The figure shows three views and two pictorial views of one solid part (mm, origin at its lowest corner). Answer the questions. A direction names the side the tool comes from. Coordinates: 2 decimals unless noted, no trailing zeros. Loops run counter-clockwise (first coordinate to the right, second up) from the corner with the lowest first, then second, coordinate; pieces in that order, holes last. Notation, with made-up numbers: (20.25, 72) -> (44.25, 72) arc R10 ccw to (44.25, 82) -> close; hole circle Ø10 at (-9, 51). An arc over 180 degrees is marked (long way). Answer as a JSON object with one key per item and string values. Group by question number.
1) Section C-C, the plane x = 34 is taken. Give the vertices of the cut face in (y, z).
2) Section D-D, the plane z = 13.75 is taken. Give the vertices of the cut face in (x, y).
3) Which of the six approach directions +Z, -Z, +X, -X, +Y, -Y give full straight-line access (tool end or side, diameter ignored) to the marked faces 1, 2 and 3?
4) Section B-B, the plane z = 4.56 is taken. Give the vertices of the cut face in (x, y), plus the area to 3 significant figures.
5) Section A-A, the plane y = 38.5 is taken. Give the vertices of the cut face in (x, z), plus the area to 3 significant figures.
6) Flat-ended cylindrical pins translate along their axes: P1, Ø8, axis at y = 24.5, z = 19.5, coming from the -X side; P2, Ø8, axis at y = 25.5, z = 11.5, coming from the +X side; P3, Ø12, axis at x = 60, z = 12, coming from the +Y side; P4, Ø1.8, axis at x = 24.81, z = 22.94, coming from the +Y side. Find the tip coordinate at first contact, or state that the pin passes through.
7) Consider probe 1 along Z at (x, y) = (43.19, 63.4); probe 2 along X at (y, z) = (62.65, 22.94); probe 3 along Z at (x, y) = (43, 63). Determine where each line is inside the solid, lowest interval first. Write a range as [from, to].
8) Determine the mould class of the marked faces 4, 5 and 6 for opening direction X: released by +X, released by -X, zero draft, split by the parting line, or undercut.
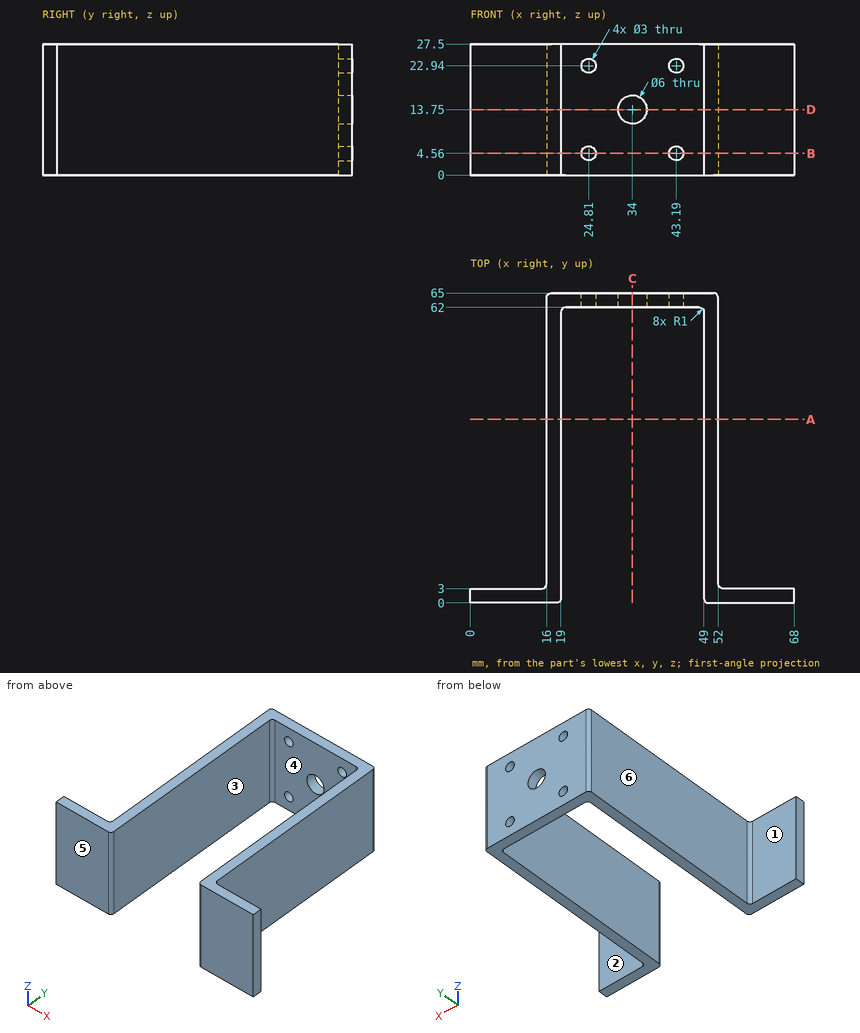
Determined:
{
 "1": {"outline": "(62, 0) -> (65, 0) -> (65, 10.75) -> (62, 10.75) -> close; (62, 16.75) -> (65, 16.75) -> (65, 27.5) -> (62, 27.5) -> close"},
 "2": {"outline": "(0, 0) -> (18, 0) arc R1 ccw to (19, 1) -> (19, 61) arc R1 cw to (20, 62) -> (31, 62) -> (31, 65) -> (17, 65) arc R1 ccw to (16, 64) -> (16, 4) arc R1 cw to (15, 3) -> (0, 3) -> close; (37, 62) -> (48, 62) arc R1 cw to (49, 61) -> (49, 1) arc R1 ccw to (50, 0) -> (68, 0) -> (68, 3) -> (53, 3) arc R1 cw to (52, 4) -> (52, 64) arc R1 ccw to (51, 65) -> (37, 65) -> close"},
 "3": {"face 1": "+Z, -Z, -X, +Y", "face 2": "+Z, -Z, +X, +Y", "face 3": "+Z, -Z, -Y"},
 "4": {"outline": "(0, 0) -> (18, 0) arc R1 ccw to (19, 1) -> (19, 61) arc R1 cw to (20, 62) -> (23.31, 62) -> (23.31, 65) -> (17, 65) arc R1 ccw to (16, 64) -> (16, 4) arc R1 cw to (15, 3) -> (0, 3) -> close; (26.31, 62) -> (41.69, 62) -> (41.69, 65) -> (26.31, 65) -> close; (44.69, 62) -> (48, 62) arc R1 cw to (49, 61) -> (49, 1) arc R1 ccw to (50, 0) -> (68, 0) -> (68, 3) -> (53, 3) arc R1 cw to (52, 4) -> (52, 64) arc R1 ccw to (51, 65) -> (44.69, 65) -> close", "area": "558 mm²"},
 "5": {"outline": "(16, 0) -> (19, 0) -> (19, 27.5) -> (16, 27.5) -> close; (49, 0) -> (52, 0) -> (52, 27.5) -> (49, 27.5) -> close", "area": "165 mm²"},
 "6": {"P1": "x = 16", "P2": "x = 52", "P3": "y = 3", "P4": "through"},
 "7": {"probe 1": "[0, 3.06], [6.06, 21.44], [24.44, 27.5]", "probe 2": "[16, 23.31], [26.31, 41.69], [44.69, 52]", "probe 3": "[0, 3.07], [6.05, 21.45], [24.43, 27.5]"},
 "8": {"face 4": "undercut", "face 5": "zero draft", "face 6": "released by -X"}
}
